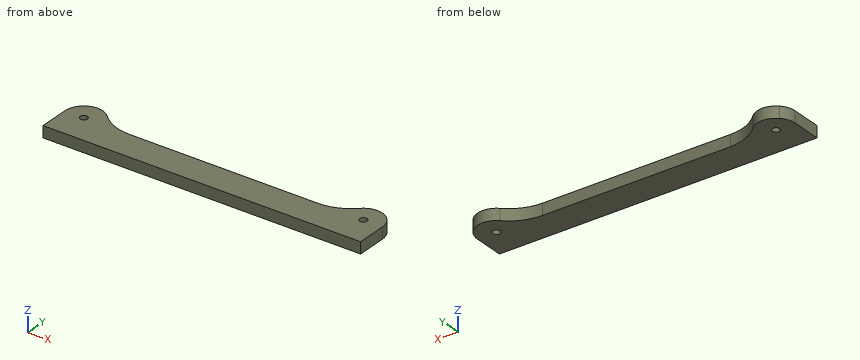
Autodesk Inventor part; units mm, degrees
ref_plane "YZ Plane" through (0, 0, 0) normal (1, 0, 0) x (0, 1, 0)
ref_plane "XZ Plane" through (0, 0, 0) normal (0, 1, 0) x (-1, 0, 0)
ref_plane "XY Plane" through (0, 0, 0) normal (0, 0, 1) x (1, 0, 0)
sketch "スケッチ2" plane through (0, 0, 0) normal (0, 0, 1) x (1, 0, 0)
  circle A0 centre (-61, -189) radius 2.1 construction
  circle A1 centre (61, -189) radius 2.1 construction
  arc A2 (66.8579, -183.1421) -> (55.1421, -183.1421) centre (61, -189) ccw
  arc A3 (41, -189) -> (55.1421, -183.1421) centre (41, -169) ccw
  line L0 (41, -189) -> (-41, -189)
  arc A4 (-55.1421, -183.1421) -> (-41, -189) centre (-41, -169) ccw
  arc A5 (-55.1421, -183.1421) -> (-66.8579, -183.1421) centre (-61, -189) ccw
  arc A6 (69.2843, -189) -> (66.8579, -183.1421) centre (61, -189) ccw
  arc A7 (-66.8579, -183.1421) -> (-69.2843, -189) centre (-61, -189) ccw
  line L1 (69.2843, -189) -> (69.2843, -202)
  line L2 (69.2843, -202) -> (-69.2843, -202)
  line L3 (-69.2843, -202) -> (-69.2843, -189)
  circle A8 centre (61, -189) radius 1.6
  circle A9 centre (-61, -189) radius 1.6
  point P0 (0, 0)
  point P1 (234, -202)
extrude "押し出し1" add sketch "スケッチ2" along normal blind 5
properties part number "radiator_adapter_02"
Geometry check sheet. Reference: the model listing, model coordinates, mm. Round coordinates to 2 decimals unless told otherwise and drop trailing zeros. Loops run counter-clockwise (first coordinate to the right, second up) from the corner with the lowest first, then second, coordinate; pieces in that order, holes last.
Item 1: Gauge pin test, flat ends, axial feed: pin 1 (12 mm diameter, centred on x = -4, y = -195, fed in from -Z); pin 2 (2.5 mm diameter, centred on x = 61, y = -189, fed in from -Z). Record the tip position at first contact, or that the pin passes through.
Item 2: Cross-section at C-C on x = -26.5. Record the boundary of the cut face in (y, z).
Item 3: Cross-section at D-D on x = -44. Record the boundary of the cut face in (y, z).
Item 4: Cross-section at A-A on z = 1.85. Record the boundary of the cut face in (x, y), then the cut area to 3 significant figures.
Item 5: Thickness scan on line 1 (Y direction, x = 61, z = 3.55); line 2 (Y direction, x = 2, z = 4.35); line 3 (X direction, y = -185.25, z = 0.85). Record the ranges inside material, lowest first.
Item 6: Cross-section at B-B on x = -61. Record the boundary of the cut face in (y, z).
Answer sheet:
1. pin 1: stops at z = 0
1. pin 2: passes through
2. outline: (-202, 0) - (-189, 0) - (-189, 5) - (-202, 5) - close
3. outline: (-202, 0) - (-188.77, 0) - (-188.77, 5) - (-202, 5) - close
4. outline: (-69.28, -202) - (69.28, -202) - (69.28, -189) arc R8.28 ccw to (66.86, -183.14) arc R8.28 ccw to (55.14, -183.14) arc R20 cw to (41, -189) - (-41, -189) arc R20 cw to (-55.14, -183.14) arc R8.28 ccw to (-66.86, -183.14) arc R8.28 ccw to (-69.28, -189) - close; hole circle Ø3.2 at (-61, -189); hole circle Ø3.2 at (61, -189)
4. area: 2,030 mm2
5. line 1: y = -202 to -190.6, -187.4 to -180.72
5. line 2: y = -202 to -189
5. line 3: x = -68.39 to -52.66, 52.66 to 68.39
6. outline: (-202, 0) - (-190.6, 0) - (-190.6, 5) - (-202, 5) - close; (-187.4, 0) - (-180.72, 0) - (-180.72, 5) - (-187.4, 5) - close
